from build123d import *

# Parameters (mm, degrees)
F1_R     = 7.5
F2_DEPTH = 3
F1_R_2   = 4.9
F3_DEPTH = 5
F4_DEPTH = 11.5


# Not quite as in the source:
# - a feature names something its author has since deleted; it is built from what else it names


with BuildPart() as f2:
    # F1 (on Top) → F2 (new body)
    with BuildSketch(Plane.XY):
        with BuildLine():
            Line((120, 10), (0, 10))
            ThreePointArc((0, 10), (-10, 0), (0, -10))
            Line((0, -10), (120, -10))
            Line((120, -10), (140, -10))
            ThreePointArc((140, -10), (150, 0), (140, 10))
            Line((140, 10), (120, 10))
        make_face()
        Circle(F1_R, mode=Mode.SUBTRACT)
        with BuildLine():
            ThreePointArc((20, -5.7), (14.3, 0), (20, 5.7))
            Line((20, 5.7), (120, 5.7))
            Line((120, 5.7), (140, 5.7))
            ThreePointArc((140, 5.7), (145.7, 0), (140, -5.7))
            Line((140, -5.7), (120, -5.7))
            Line((120, -5.7), (20, -5.7))
        make_face(mode=Mode.SUBTRACT)
    extrude(amount=F2_DEPTH)

    # F1 (on Top) → F3 (join)
    with BuildSketch(Plane.XY):
        Circle(F1_R)
        Circle(F1_R_2, mode=Mode.SUBTRACT)
    extrude(amount=F3_DEPTH)

    # F1 (on Top) → F4 (join)
    with BuildSketch(Plane.XY):
        Circle(F1_R_2)
        with BuildLine():
            Line((2.2847319318, -2.45), (0, -2.45))
            Line((0, -2.45), (-2.2847319318, -2.45))
            ThreePointArc((-2.2847319318, -2.45), (-3.35, 0), (-2.2847319318, 2.45))
            Line((-2.2847319318, 2.45), (0, 2.45))
            Line((0, 2.45), (2.2847319318, 2.45))
            ThreePointArc((2.2847319318, 2.45), (3.35, 0), (2.2847319318, -2.45))
        make_face(mode=Mode.SUBTRACT)
    extrude(amount=F4_DEPTH)

    # F6 (on plane+point) → F7 (revolve)
    with BuildSketch(Plane.XZ):
        Polygon((5.15, 10.75), (4.9, 11.5), (4.9, 10), align=None)
    revolve(axis=Axis((0, 0, 5.75), (0, 0, 1)))


solid = f2.part
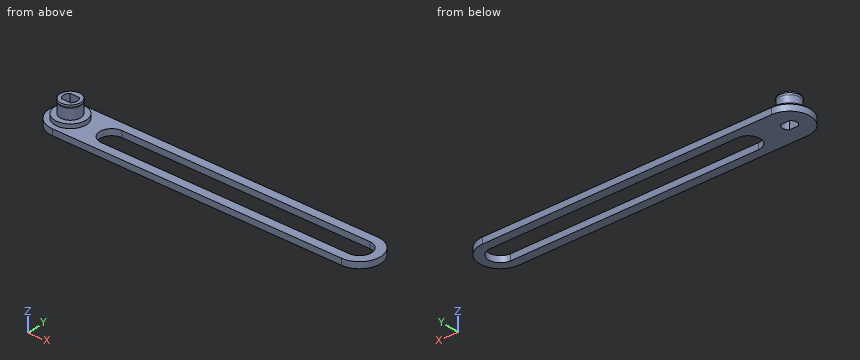
Can you work these out from the model? Positions are in its coordinate system, mm. Give positions to 0.01 mm unless a question says otherwise; leave off trailing zeros. Write each loop counter-clockwise with the first axis right and the second up, starting at its lowest first coordinate (ties: lowest second). Pieces come first, ordered by that corner, then holes. Notation, with made-up numbers: (82, 26.5) -> (114, 26.5) arc R13 ccw to (114, 45.5) -> close; hole circle Ø6 at (59, 16.5). An arc over 180 degrees is marked (long way). Answer as a JSON object with one key per item and string values. Group by question number.
Item 1: Suppose I cut it at A-A (x = 88). Please give me the cut outline in (y, z).
Item 2: I'm going to push flat-ended pins straight in: P1, Ø8, axis at x = 11.5, y = 2.5, coming from the +Z side; P2, Ø3.5, axis at x = 1, z = 4, coming from the +Y side; P3, Ø2.5, axis at x = 0, z = 6.5, coming from the -Y side. Where does each tip first touch, or does it pass through?
Item 3: Suppose I cut it at B-B (y = 0). Please give me the cut outline in (x, z), plus the area to 3 significant figures.
Item 4: Please list where these lines run through material, in increasing order: line 1 (Y direction, x = 73, z = 1); line 2 (X direction, y = 1.75, z = 1); line 3 (X direction, y = -4.25, z = 8.75). Write a range as [from, to].
Item 5: Suppose I cut it at C-C (z = 1.5). Please give me the cut outline in (x, y), plus the area to 3 significant figures.
Item 6: Suppose I cut it at D-D (z = 7.5). Please give me the cut outline in (x, y), plus the area to 3 significant figures.
Findings:
{
 "1": {"outline": "(-10, 0) -> (-5.7, 0) -> (-5.7, 3) -> (-10, 3) -> close; (5.7, 0) -> (10, 0) -> (10, 3) -> (5.7, 3) -> close"},
 "2": {"P1": "stops at z = 3", "P2": "stops at y = 10", "P3": "stops at y = -4.9"},
 "3": {"outline": "(-10, 0) -> (-3.35, 0) -> (-3.35, 11.5) -> (-4.9, 11.5) -> (-5.15, 10.75) -> (-4.9, 10) -> (-4.9, 5) -> (-7.5, 5) -> (-7.5, 3) -> (-10, 3) -> close; (3.35, 0) -> (14.3, 0) -> (14.3, 3) -> (7.5, 3) -> (7.5, 5) -> (4.9, 5) -> (4.9, 10) -> (5.15, 10.75) -> (4.9, 11.5) -> (3.35, 11.5) -> close; (145.7, 0) -> (150, 0) -> (150, 3) -> (145.7, 3) -> close", "area": "103 mm²"},
 "4": {"line 1": "y = [-10, -5.7], [5.7, 10]", "line 2": "x = [-9.85, -2.86], [2.86, 14.58], [145.42, 149.85]", "line 3": "x = [-2.44, 2.44]"},
 "5": {"outline": "(0, -10) -> (140, -10) arc R10 ccw to (140, 10) -> (0, 10) arc R10 ccw to start; hole (-2.28, -2.45) -> (2.28, -2.45) arc R3.35 ccw to (2.28, 2.45) -> (-2.28, 2.45) arc R3.35 ccw to start; hole (20, -5.7) -> (140, -5.7) arc R5.7 ccw to (140, 5.7) -> (20, 5.7) arc R5.7 ccw to start", "area": "1,610 mm²"},
 "6": {"outline": "circle Ø9.8 at (0, 0); hole (-2.28, -2.45) -> (2.28, -2.45) arc R3.35 ccw to (2.28, 2.45) -> (-2.28, 2.45) arc R3.35 ccw to start", "area": "45.8 mm²"}
}
